Part model, mm, in its own coordinate system. A direction names the side the tool comes from. Coordinates: 2 decimals unless noted, no trailing zeros. Write each loop counter-clockwise with the first axis right and the second up, starting at its lowest first coordinate (ties: lowest second). Pieces come first, ordered by that corner, then holes. Notation, with made-up numbers: (24.5, -27) -> (72.5, -27) arc R20 ccw to (72.5, -12) -> close; hole circle Ø8 at (11.25, 83.25). An arc over 180 degrees is marked (long way). One line per question, with ' | ' between items. Start each with the question number.
Item 1: Pin check, flat tips, straight feed: pin 1 (2.5 mm diameter, centred on y = 5, z = -3, fed in from -X); pin 2 (5 mm diameter, centred on x = 32.5, y = 2.5, fed in from +Z); pin 3 (0.6 mm diameter, centred on y = 6, z = -18, fed in from -X). Stop position of each tip, or through.
Item 2: Saw through at B-B (x = 56). List the corners of the cut face in (y, z), and give its area (3 significant figures).
Item 3: Saw through at A-A (z = -7). List the corners of the cut face in (x, y), and give its area (3 significant figures).
Item 4: Probe probe 1 along X at (y, z) = (5, -7); probe 2 along X at (y, z) = (1.15, -3); probe 3 along X at (y, z) = (6.5, -11.5). List the from-to ranges inside material, lowest first. Write a range as [from, to].
Item 5: Two-plate mould, pull along Y, no slides. Class faces 1 (the cylindrical face through (8.806, 4.944, 20.7)), 2 (the flat face through (29, 10, -2)), 3 (the flat face through (46, 7, -2)): pulls with the +Y half, pulls with the -Y half, needs draft (parallel to the pull), parting line crosses it, or undercut.
Item 6: 3-axis set-ups, long thin cutter, end or side, ignore diameter. For faces 4 (the flat face through (59.025, 5, -18)), 5 (the cylindrical face through (12.84, 5.07, -14.1)), 6 (the flat face through (46, 2, -2)): which of +Z, -Z, +X, -X, +Y, -Y reach the whole face in a straight line?
from build123d import *

# Parameters (mm, degrees)
CROQUIS1_R              = 1.5
SALIENTE_EXTRUIR1_DEPTH = 10
REDONDEO1_R             = 3
CROQUIS3_R              = 1.5
CORTAR_EXTRUIR2_DEPTH   = 11
REDONDEO2_R             = 5
CROQUIS4_W              = 6
CROQUIS4_H              = 5
CORTAR_EXTRUIR3_DEPTH   = 6
REDONDEO3_R             = 1


with BuildPart() as part:
    # Croquis1 → Saliente-Extruir1 (new body)
    with BuildSketch(Plane(origin=(0, 0, 0), x_dir=(1, 0, 0), z_dir=(0, 1, 0))):
        with BuildLine():
            Line((13.699946153, 11.735059562), (59.024625957, 11.735059562))
            Line((59.024625957, 11.735059562), (59.024625957, 18.735059562))
            Line((59.024625957, 18.735059562), (67.731133792, 18.735059562))
            Line((67.731133792, 18.735059562), (67.731133792, 0))
            Line((67.731133792, 0), (17.731133792, 0))
            ThreePointArc((17.731133792, 0), (9.262538254, -20.305782945), (-11.922145642, -26.243046592))
            ThreePointArc((-11.922145642, -26.243046592), (-1.979394551, -14.930389049), (0, 0))
            Line((0, 0), (0, 15))
            Line((0, 15), (13.699946153, 15))
            Line((13.699946153, 15), (13.699946153, 11.735059562))
        make_face()
        with Locations(Location((8, 7, 0), (0, 0, 270))):
            Circle(CROQUIS1_R, mode=Mode.SUBTRACT)
    extrude(amount=SALIENTE_EXTRUIR1_DEPTH)

    # Redondeo1
    redondeo1_edges = [part.edges().sort_by_distance(p)[0] for p in [
        (0, 5, -15),
        (13.699946153, 5, -15),
    ]]
    fillet(redondeo1_edges, radius=REDONDEO1_R)

    # Croquis3 → Cortar-Extruir2 (cut)
    with BuildSketch(Plane(origin=(0, 10, 0), x_dir=(1, 0, 0), z_dir=(0, 1, 0))):
        with Locations(Location((47.731133792, 3, 0), (0, 0, 270))):
            Circle(CROQUIS3_R)
    extrude(amount=-CORTAR_EXTRUIR2_DEPTH, mode=Mode.SUBTRACT)

    # Redondeo2
    redondeo2_edges = [part.edges().sort_by_distance(p)[0] for p in [
        (67.731133792, 5, 0),
        (17.731133792, 5, 0),
        (59.024625957, 5, -11.735059562),
    ]]
    fillet(redondeo2_edges, radius=REDONDEO2_R)

    # Croquis4 → Cortar-Extruir3 (cut)
    with BuildSketch(Plane.XY):
        with Locations((47.731133792, 4.5)):
            Rectangle(CROQUIS4_W, CROQUIS4_H)
    extrude(amount=-CORTAR_EXTRUIR3_DEPTH, mode=Mode.SUBTRACT)

    # Redondeo3
    redondeo3_edges = [part.edges().sort_by_distance(p)[0] for p in [
        (7.547710992, 0, 21.694525169),
        (-1.979394551, 0, 14.930389049),
        (-11.922145642, 5, 26.243046592),
        (0, 5, 0),
        (-1.979394551, 10, 14.930389049),
        (7.547710992, 10, 21.694525169),
        (67.731133792, 0, -11.867529781),
        (67.731133792, 10, -11.867529781),
        (42.644255321, 0, 0),
        (66.266667698, 0, -1.464466094),
        (42.644255321, 10, 0),
        (66.266667698, 10, -1.464466094),
        (19.238162868, 0, 1.260639287),
        (19.238162868, 10, 1.260639287),
    ]]
    fillet(redondeo3_edges, radius=REDONDEO3_R)


solid = part.part
From the geometry:
1) pin 1: x = 0 | pin 2: z = 0 | pin 3: x = 59.02
2) outline: (0, -12.14) -> (10, -12.14) -> (10, -1) arc R1 ccw to (9, 0) -> (1, 0) arc R1 ccw to (0, -1) -> close | area: 121 mm2
3) outline: (0, 0) -> (6.5, 0) -> (6.5, 10) -> (0, 10) -> close; (9.5, 0) -> (66.73, 0) arc R1 ccw to (67.73, 1) -> (67.73, 9) arc R1 ccw to (66.73, 10) -> (9.5, 10) -> close | area: 647 mm2
4) probe 1: [0, 6.5], [9.5, 67.73] | probe 2: [0, 46.23], [49.23, 67.31] | probe 3: [0, 67.73]
5) face 1: needs draft | face 2: pulls with the +Y half | face 3: undercut
6) face 4: -Z, -X, +Y, -Y | face 5: -Z, +Y, -Y | face 6: +Z
